from build123d import *

# Parameters (mm, degrees)
SKETCH1_R           = 7.5
BOSS_EXTRUDE1_DEPTH = 10
SKETCH5_R           = 6
BOSS_EXTRUDE2_DEPTH = 2
FILLET2_R           = 1
BOSS_EXTRUDE3_DEPTH = 6
CUT_EXTRUDE4_DEPTH  = 29
CUT_EXTRUDE5_START  = -1
SKETCH10_R          = 2
CUT_EXTRUDE5_DEPTH  = 20


with BuildPart() as part:
    # Sketch1 → Boss-Extrude1 (new body)
    with BuildSketch(Plane(origin=(0, 0, 0), x_dir=(1, 0, 0), z_dir=(0, 1, 0))):
        with Locations(Location((0, 0, 0), (0, 0, 270))):
            Circle(SKETCH1_R)
    boss_extrude1 = extrude(amount=BOSS_EXTRUDE1_DEPTH)

    # Sketch5 → Boss-Extrude2 (add)
    with BuildSketch(Plane(origin=(0, 10, 0), x_dir=(1, 0, 0), z_dir=(0, 1, 0))):
        with Locations(Location((0, 0, 0), (0, 0, 270))):
            Circle(SKETCH5_R)
    boss_extrude2 = extrude(amount=BOSS_EXTRUDE2_DEPTH)

    # Fillet2
    fillet2_edges = [part.edges().sort_by_distance(p)[0] for p in [
        (0, 10, -6),
    ]]
    fillet(fillet2_edges, radius=FILLET2_R)

    # Sketch6 → Boss-Extrude3 (add, symmetric)
    with BuildSketch(Plane(origin=(0, 0, 0), x_dir=(0, 0, -1), z_dir=(1, 0, 0))):
        Polygon((6, 12), (-6, 12), (-11, 12), (-11, 27), (-9, 27), (-9, 14), (9, 14), (9, 27), (11, 27), (11, 12), align=None)
    boss_extrude3 = extrude(amount=BOSS_EXTRUDE3_DEPTH, both=True)

    # Sketch9 → Cut-Extrude4 (cut)
    with BuildSketch(Plane.XY.offset(11)):
        with BuildLine():
            Line((-6, 27), (-6, 21))
            ThreePointArc((-6, 21), (-4.052343178, 25.052343178), (0, 27))
            Line((0, 27), (-6, 27))
        make_face()
        with BuildLine():
            ThreePointArc((0, 27), (4.052343178, 25.052343178), (6, 21))
            Line((6, 21), (6, 27))
            Line((6, 27), (0, 27))
        make_face()
    cut_extrude4 = extrude(amount=-CUT_EXTRUDE4_DEPTH, mode=Mode.SUBTRACT)

    # Sketch10 → Cut-Extrude5 (cut)
    with BuildSketch(Plane(origin=(0, 0, 9), x_dir=(-1, 0, 0), z_dir=(0, 0, -1)).offset(CUT_EXTRUDE5_START)):
        with Locations(Location((0, 24.25, 0), (0, 0, 180))):
            Circle(SKETCH10_R)
    cut_extrude5 = extrude(amount=CUT_EXTRUDE5_DEPTH, mode=Mode.SUBTRACT)

    # Mirror2: Boss-Extrude1 across plane
    add(boss_extrude1.mirror(Plane.ZX))

    # Mirror9: Boss-Extrude2, Boss-Extrude3 across plane
    add(boss_extrude2.mirror(Plane.ZX))
    add(boss_extrude3.mirror(Plane.ZX))

    # Mirror11: Cut-Extrude4, Cut-Extrude5 across plane
    add(cut_extrude4.mirror(Plane.ZX), mode=Mode.SUBTRACT)
    add(cut_extrude5.mirror(Plane.ZX), mode=Mode.SUBTRACT)


solid = part.part
The listing builds one solid part. Answer for the finished solid, in the listing's coordinates (mm). A direction names the side the tool comes from. Coordinates: 2 decimals unless noted, no trailing zeros. Write each loop counter-clockwise with the first axis right and the second up, starting at its lowest first coordinate (ties: lowest second). Pieces come first, ordered by that corner, then holes. Notation, with made-up numbers: M -3.75,77 L 20.25,77 A18 ccw 20.25,85 Z; hole C -11.5,42 d4. An arc over 180 degrees is marked long. Write each question's results on one line, items separated by ' | '.
Item 1: The part is cut by section B-B on y = 8. Determine the outline of the cut face in (x, z), and give its area (3 significant figures).
Answer below:
outline: C 0,0 d15 | area: 177 mm2
Item 2: Consider probe 1 along Z at (x, y) = (-5, 22.5); probe 2 along Y at (x, z) = (2.5, 3.75); probe 3 along Y at (x, z) = (-4, -9.75). Determine where each line is inside the solid, lowest interval first. Write a range as [from, to].
Answer below:
probe 1: [-11, -9], [9, 11] | probe 2: [-14, 14] | probe 3: [-25.1, -12], [12, 25.1]
Item 3: Which of the six approach directions +Z, -Z, +X, -X, +Y, -Y give full straight-line access (tool end or side, diameter ignored) to faces 5 (the face through (-7, 10, -2)), 6 (the face through (0, -19, 9)), 7 (the face through (0, 19, 9))?
Answer below:
face 5: none | face 6: +X, -X, -Y | face 7: +X, -X, +Y
Item 4: Given P1, Ø7, axis at y = -15.5, z = -1, coming from the +X side; P2, Ø2.5, axis at y = -15, z = -3.5, coming from the -X side; P3, Ø4, axis at x = 3, y = 7, coming from the -Z side, each flat-ended and moving along its own axis, determine where each tip first touches the part or whether it passes through.
Answer below:
P1: x = 6 | P2: x = -6 | P3: z = -7.43
Item 5: For a pull along Z with two mould halves and no side action, classify faces 1 (the face through (0, 19, 11)), 2 (the face through (0, -20, -11)), 3 (the face through (0, -19, -9)), 4 (the face through (4.007, -25.097, -9.986)) as released by +Z, released by -Z, zero draft, split by the parting line, or undercut.
Answer below:
face 1: released by +Z | face 2: released by -Z | face 3: undercut | face 4: zero draft
Item 6: The part is cut by section A-A on y = 19. Determine the outline of the cut face in (x, z).
Answer below:
outline: M -6,-11 L 6,-11 L 6,-9 L -6,-9 Z; M -6,9 L 6,9 L 6,11 L -6,11 Z
